```python
from build123d import *

# Parameters (mm, degrees)
EXTRUDE_1_DEPTH     = 3
SKETCH_2_R          = 6.5
SKETCH_2_W          = 25
SKETCH_2_H          = 15
CUT_EXTRUDE_1_DEPTH = 57.207205944


with BuildPart() as part:
    # 草图1 → 凸台-拉伸1 (new body)
    with BuildSketch(Plane(origin=(0, 0, 0), x_dir=(1, 0, 0), z_dir=(0, 1, 0))):
        Polygon((-50, -22.5), (-40, -22.5), (-40, -25.5), (-25, -25.5), (-25, -22.5), (-7.5, -22.5), (-7.5, -25.5), (7.5, -25.5), (7.5, -22.5), (25, -22.5), (25, -25.5), (40, -25.5), (40, -22.5), (50, -22.5), (50, -17.5), (47, -17.5), (47, -7.5), (50, -7.5), (50, 7.5), (47, 7.5), (47, 17.5), (50, 17.5), (50, 22.5), (40, 22.5), (40, 25.5), (25, 25.5), (25, 22.5), (7.5, 22.5), (7.5, 25.5), (-7.5, 25.5), (-7.5, 22.5), (-25, 22.5), (-25, 25.5), (-40, 25.5), (-40, 22.5), (-50, 22.5), (-50, 17.5), (-47, 17.5), (-47, 7.5), (-50, 7.5), (-50, -7.5), (-47, -7.5), (-47, -17.5), (-50, -17.5), align=None)
    extrude(amount=EXTRUDE_1_DEPTH)

    # 草图2 → 切除-拉伸1 (cut, through all)
    with BuildSketch(Plane(origin=(0, 3, 0), x_dir=(1, 0, 0), z_dir=(0, 1, 0))):
        with Locations(Location((-31, 2.5, 0), (0, 0, 270))):
            Circle(SKETCH_2_R)
        with Locations((19, -9)):
            Rectangle(SKETCH_2_W, SKETCH_2_H)
    extrude(amount=-CUT_EXTRUDE_1_DEPTH, mode=Mode.SUBTRACT)


solid = part.part
```
Source: CAD feature listing. Evaluate the final solid. Frame: model axes, mm. A direction names the side the tool comes from. Round coordinates to 2 decimals unless told otherwise and drop trailing zeros. Loops run counter-clockwise (first coordinate to the right, second up) from the corner with the lowest first, then second, coordinate; pieces in that order, holes last.
(1) Section query B-B (z = -2.5). Output: boundary loops of the cut face in (x, y), and give its area (3 significant figures).
From the geometry:
outline: (-50, 0) - (-37.5, 0) - (-37.5, 3) - (-50, 3) - close; (-24.5, 0) - (50, 0) - (50, 3) - (-24.5, 3) - close
area: 261 mm2
(2) Section query A-A (x = 18). Output: boundary loops of the cut face in (y, z), and give its area (3 significant figures).
From the geometry:
outline: (0, -22.5) - (3, -22.5) - (3, 1.5) - (0, 1.5) - close; (0, 16.5) - (3, 16.5) - (3, 22.5) - (0, 22.5) - close
area: 90.0 mm2
(3) Section query D-D (x = -44). Output: boundary loops of the cut face in (y, z).
From the geometry:
outline: (0, -22.5) - (3, -22.5) - (3, 22.5) - (0, 22.5) - close
(4) Material intervals for probe 1 along X at (y, z) = (2.05, -2.5); probe 2 along X at (y, z) = (0.25, 16); probe 3 along Z at (x, y) = (25.5, 2.1), sorted ascending.
From the geometry:
probe 1: x = -50 to -37.5, -24.5 to 50
probe 2: x = -47 to 6.5, 31.5 to 47
probe 3: z = -25.5 to 1.5, 16.5 to 25.5
(5) Contact query for flat-ended pins moving along their axis: pin 1 Ø0.9 at (y, z) = (1.5, -24) entering from -X; pin 2 Ø0.9 at (y, z) = (1, 11) entering from -X; pin 3 Ø1.5 at (x, y) = (45.5, 1) entering from +Z. Output: stop coordinate, or through.
From the geometry:
pin 1: stops at x = -40
pin 2: stops at x = -47
pin 3: stops at z = 22.5
(6) Section query C-C (y = 1.95). Give the number of separate pieces and of enclosed holes in the cut face, and give its area (3 significant figures).
From the geometry:
separate pieces: 1
enclosed holes: 2
area: 4,140 mm2
(7) Pull-direction query (X, two-part tool) for faces 4 (the flat face through (-7.5, 1, -24)), 5 (the flat face through (0, 1, 25.5)), 6 (the flat face through (-50, 1, -20)); classes: +X half, -X half, draft (parallel to the pull), parting line (faces both ways), or undercut.
From the geometry:
face 4: undercut
face 5: draft
face 6: -X half
(8) Access query for faces 1 (the flat face through (-7.5, 1, 24)), 2 (the flat face through (-45, 1, 22.5)), 3 (the flat face through (47, 1, -12)). Directions: +Z, -Z, +X, -X, +Y, -Y. A direction counts if a zero-diameter tool reaches every point of the face in a straight line with its end or side. Return the directions, or none.
From the geometry:
face 1: +Z, +Y, -Y
face 2: +Z, -X, +Y, -Y
face 3: +X, +Y, -Y
